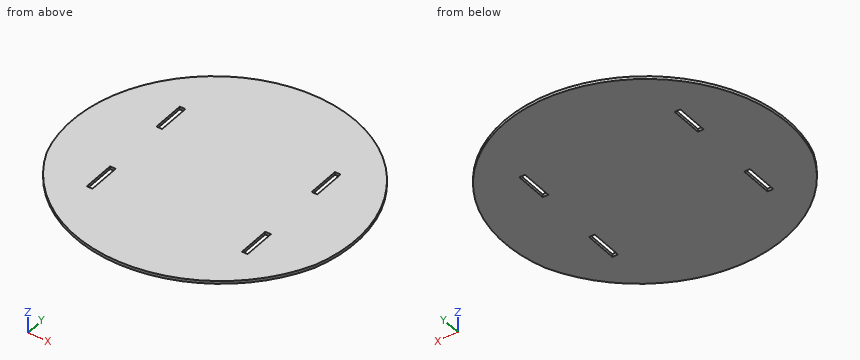
```python
from build123d import *

# Parameters (mm, degrees)
ESBO_O1_W                = 6
ESBO_O1_H                = 35
RESSALTO_EXTRUS_O1_DEPTH = 3


with BuildPart() as part:
    # Esboço1 → Ressalto-extrusão1 (new body)
    with BuildSketch(Plane.XY):
        with BuildLine():
            ThreePointArc((141.421356237, -50), (0, 150), (-141.421356237, -50))
            ThreePointArc((-141.421356237, -50), (0, -142.957457878), (141.421356237, -50))
        make_face()
        with Locations((-82, -52.5)):
            Rectangle(ESBO_O1_W, ESBO_O1_H, mode=Mode.SUBTRACT)
        with Locations((-82, 52.5)):
            Rectangle(ESBO_O1_W, ESBO_O1_H, mode=Mode.SUBTRACT)
        with Locations((82, -52.5)):
            Rectangle(ESBO_O1_W, ESBO_O1_H, mode=Mode.SUBTRACT)
        with Locations((82, 52.5)):
            Rectangle(ESBO_O1_W, ESBO_O1_H, mode=Mode.SUBTRACT)
    extrude(amount=RESSALTO_EXTRUS_O1_DEPTH)


solid = part.part
```
The model under review builds one solid part; all positions refer to its coordinate system, in mm. Round coordinates to 2 decimals unless told otherwise and drop trailing zeros. Write each loop counter-clockwise with the first axis right and the second up, starting at its lowest first coordinate (ties: lowest second). Pieces come first, ordered by that corner, then holes.
(1) We need section B-B on y = -64. Give the boundary of the cut face in (x, z).
(2) We need section C-C on x = -114. Give the boundary of the cut face in (y, z).
(3) Wall thickness on L1, parallel to X at y = 39, z = 0.6; L2, parallel to X at y = 50.5, z = 0.7; L3, parallel to X at y = -86.5, z = 0.55: over which ranges is each line inside the solid? List them lowest first.
(4) We need section D-D on y = -112.5. Give the boundary of the cut face in (x, z).
(5) We need section A-A on z = 1.85. Give the boundary of the cut face in (x, y).
(6) Insertion check: pin 1 (1.5 mm diameter, centred on y = 53, z = 1, fed in from -X); pin 2 (0.9 mm diameter, centred on y = -47.5, z = 2, fed in from -X); pin 3 (1.5 mm diameter, centred on x = -82, z = 2, fed in from +Y). Each pin has a flat end and moves straight along its axis. Give the tip position at first contact, or say it passes through.
Findings below:
1. outline: (-134.51, 0) - (-85, 0) - (-85, 3) - (-134.51, 3) - close; (-79, 0) - (79, 0) - (79, 3) - (-79, 3) - close; (85, 0) - (134.51, 0) - (134.51, 3) - (85, 3) - close
2. outline: (-92.52, 0) - (97.49, 0) - (97.49, 3) - (-92.52, 3) - close
3. L1: x = -144.84 to -85, -79 to 79, 85 to 144.84
3. L2: x = -141.24 to -85, -79 to 79, 85 to 141.24
3. L3: x = -119.2 to 119.2
4. outline: (-91.96, 0) - (91.96, 0) - (91.96, 3) - (-91.96, 3) - close
5. outline: (-141.42, -50) arc R154.05 ccw to (141.42, -50) arc R150 ccw (long way) to start; hole (-85, -70) - (-79, -70) - (-79, -35) - (-85, -35) - close; hole (-85, 35) - (-79, 35) - (-79, 70) - (-85, 70) - close; hole (79, -70) - (85, -70) - (85, -35) - (79, -35) - close; hole (79, 35) - (85, 35) - (85, 70) - (79, 70) - close
6. pin 1: stops at x = -140.61
6. pin 2: stops at x = -142.43
6. pin 3: stops at y = 126.09
